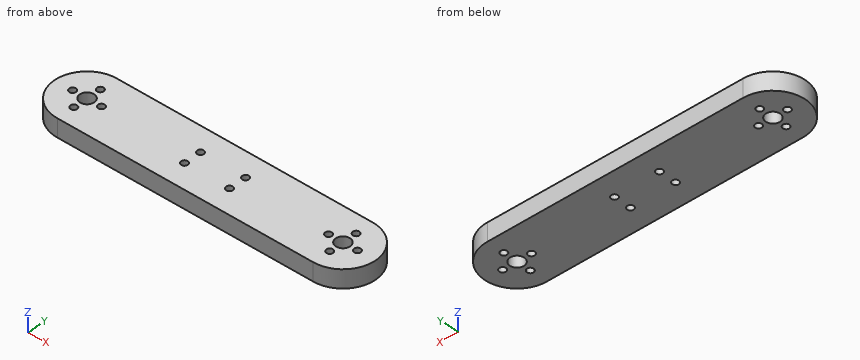
from build123d import *

# Parameters (mm, degrees)
F0_R     = 1.85
F0_R_2   = 4
F1_DEPTH = 10


with BuildPart() as f1:
    # F0 (on Top) → F1 (new body)
    with BuildSketch(Plane.XY):
        with BuildLine():
            Line((-71, -18), (71, -18))
            ThreePointArc((71, -18), (89, 0), (71, 18))
            Line((71, 18), (-71, 18))
            ThreePointArc((-71, 18), (-89, 0), (-71, -18))
        make_face()
        with BuildLine():
            ThreePointArc((-71, -6.15), (-69.691852, -6.691852), (-69.15, -8))
            ThreePointArc((-69.15, -8), (-69.691852, -9.308148), (-71, -9.85))
            ThreePointArc((-71, -9.85), (-72.85, -8), (-71, -6.15))
        make_face(mode=Mode.SUBTRACT)
        with Locations((-12.5, -4.85)):
            Circle(F0_R, mode=Mode.SUBTRACT)
        with Locations((12.5, -4.85)):
            Circle(F0_R, mode=Mode.SUBTRACT)
        with BuildLine():
            ThreePointArc((71, -6.15), (72.308148, -6.691852), (72.85, -8))
            ThreePointArc((72.85, -8), (72.308148, -9.308148), (71, -9.85))
            ThreePointArc((71, -9.85), (69.15, -8), (71, -6.15))
        make_face(mode=Mode.SUBTRACT)
        with Locations((-79, 0)):
            Circle(F0_R, mode=Mode.SUBTRACT)
        with Locations((-71, 0)):
            Circle(F0_R_2, mode=Mode.SUBTRACT)
        with Locations((-63, 0)):
            Circle(F0_R, mode=Mode.SUBTRACT)
        with BuildLine():
            ThreePointArc((-71, 9.85), (-69.691852, 9.308148), (-69.15, 8))
            ThreePointArc((-69.15, 8), (-69.691852, 6.691852), (-71, 6.15))
            ThreePointArc((-71, 6.15), (-72.85, 8), (-71, 9.85))
        make_face(mode=Mode.SUBTRACT)
        with Locations((-12.5, 4.85)):
            Circle(F0_R, mode=Mode.SUBTRACT)
        with Locations((12.5, 4.85)):
            Circle(F0_R, mode=Mode.SUBTRACT)
        with Locations((63, 0)):
            Circle(F0_R, mode=Mode.SUBTRACT)
        with Locations((71, 0)):
            Circle(F0_R_2, mode=Mode.SUBTRACT)
        with Locations((79, 0)):
            Circle(F0_R, mode=Mode.SUBTRACT)
        with BuildLine():
            ThreePointArc((71, 9.85), (72.308148, 9.308148), (72.85, 8))
            ThreePointArc((72.85, 8), (72.308148, 6.691852), (71, 6.15))
            ThreePointArc((71, 6.15), (69.15, 8), (71, 9.85))
        make_face(mode=Mode.SUBTRACT)
    extrude(amount=F1_DEPTH)


solid = f1.part
Here's how the part is built. I have some questions about the finished solid (model axes, mm). Round coordinates to 2 decimals unless told otherwise and drop trailing zeros. Order: outer loops, then holes, each group sorted by start corner. A loop starts at its lowest first (then second) coordinate and runs counter-clockwise, first axis right, second up. Notation, with made-up numbers: M -22.75,0.25 L 5.25,0.25 A33 ccw 5.25,34.25 Z; hole C -4,54.25 d2. An arc over 180 degrees is marked long. Return JSON: item names as keys, results as strings. Group by question number.
1. If we section it at A-A on x = -63: List the corners of the cut face in (y, z) for me, then the cut area to 3 significant figures.
2. If we section it at D-D on x = 12.5: List the corners of the cut face in (y, z) for me, then the cut area to 3 significant figures.
3. I'm going to push flat-ended pins straight in: pin 1 Ø1.5 at (y, z) = (9.5, 5.5) entering from +X; pin 2 Ø3 at (x, y) = (79, 0) entering from +Z; pin 3 Ø2 at (y, z) = (7, 7.5) entering from +X; pin 4 Ø3 at (y, z) = (-4, 9) entering from +X. Where does each tip first touch, or does it pass through?
4. Please list where these lines run through material, in increasing order: probe 1 along Y at (x, z) = (-71, 6); probe 2 along Y at (x, z) = (12.5, 6.75); probe 3 along Y at (x, z) = (-63, 3.25).
5. If we section it at C-C on y = 0: List the corners of the cut face in (x, z) for me.
6. If we section it at B-B on z = 2.5: State how many separate pieces and enclosed holes the cut face has, then the cut area to 3 significant figures.
Reply:
{
 "1": {"outline": "M -18,0 L -1.85,0 L -1.85,10 L -18,10 Z; M 1.85,0 L 18,0 L 18,10 L 1.85,10 Z", "area": "323 mm^2"},
 "2": {"outline": "M -18,0 L -6.7,0 L -6.7,10 L -18,10 Z; M -3,0 L 3,0 L 3,10 L -3,10 Z; M 6.7,0 L 18,0 L 18,10 L 6.7,10 Z", "area": "286 mm^2"},
 "3": {"pin 1": "x = 86.73", "pin 2": "through", "pin 3": "x = 87.97", "pin 4": "x = 88.83"},
 "4": {"probe 1": "-18 to -9.85, -6.15 to -4, 4 to 6.15, 9.85 to 18", "probe 2": "-18 to -6.7, -3 to 3, 6.7 to 18", "probe 3": "-18 to -1.85, 1.85 to 18"},
 "5": {"outline": "M -89,0 L -80.85,0 L -80.85,10 L -89,10 Z; M -77.15,0 L -75,0 L -75,10 L -77.15,10 Z; M -67,0 L -64.85,0 L -64.85,10 L -67,10 Z; M -61.15,0 L 61.15,0 L 61.15,10 L -61.15,10 Z; M 64.85,0 L 67,0 L 67,10 L 64.85,10 Z; M 75,0 L 77.15,0 L 77.15,10 L 75,10 Z; M 80.85,0 L 89,0 L 89,10 L 80.85,10 Z"},
 "6": {"separate pieces": "1", "enclosed holes": "14", "area": "5,900 mm^2"}
}
